Autodesk Inventor part; units mm, degrees
ref_plane "YZ Plane" through (0, 0, 0) normal (1, 0, 0) x (0, 1, 0)
ref_plane "XZ Plane" through (0, 0, 0) normal (0, 1, 0) x (-1, 0, 0)
ref_plane "XY Plane" through (0, 0, 0) normal (0, 0, 1) x (1, 0, 0)
sketch "Sketch1" plane through (0, 0, 0) normal (0, 0, 1) x (1, 0, 0)
  line L0 (0, 0) -> (100, 0)
  line L1 (100, 0) -> (100, 40)
  line L2 (100, 40) -> (0, 40)
  line L3 (0, 40) -> (0, 0)
  dimension "d0" = 100
  dimension "d1" = 40
extrude "Extrusion1" add sketch "Sketch1" along normal mid plane 40
sketch "Sketch2" plane through (100, 0, 20) normal (1, 0, 0) x (0, 0, -1)
  line L0 (40, 40) -> (0, 40)
  circle A0 centre (20, 20) radius 18
  point P0 (20, 0)
  dimension "d5" = 36
extrude "Extrusion2" add sketch "Sketch2" along normal blind 80
thread "Thread1"
chamfer "Chamfer1" distance 2 angle 45 1 edges at (180, 20, 18)
sketch "Sketch3" plane through (0, 0, 20) normal (0, 0, 1) x (1, 0, 0)
  line L0 (0, 0) -> (100, 0)
  line L1 (100, 40) -> (0, 40)
  circle A0 centre (20, 20) radius 7.5
  circle A1 centre (20, 20) radius 12.5
  line L2 (100, 0) -> (100, 40)
  dimension "d13" = 80
  dimension "d14" = 15
  dimension "d15" = 25
hole "Hole1" at (20, 20, 20) direction (0, 0, -1) diameter 15 end through all counterbore diameter 25 counterbore depth 5
fillet "Fillet1" radius 20 1 edges at (0, 40, 0)
fillet "Fillet2" radius 20 1 edges at (0, 0, 0)
sketch "Sketch9" plane through (100, 40, 20) normal (0, 1, 0) x (1, 0, 0)
  line L0 (0, 0) -> (-80, 0)
  line L1 (-28, 0) -> (-28, 39.5262)
  line L2 (0, 40) -> (0, 0)
  line L3 (-108, 28) -> (-28, 28)
  line L4 (-28, 28) -> (-28, 12)
  line L5 (-28, 12) -> (-108, 12)
  line L6 (-108, 12) -> (-108, 28)
  line L7 (-80, 40) -> (0, 40)
  circle A0 centre (-28, 20) radius 8
  point P0 (-100, 20)
  point P1 (-68, 12)
  point P2 (-28, 12)
  point P3 (-28, 28)
  dimension "d37" = 28
  dimension "d38" = 0
  dimension "d39" = 12
  dimension "d40" = 16
  dimension "d41" = 16
  dimension "d42" = 80
  dimension "d43" = 16
extrude "Extrusion5" cut sketch "Sketch9" against normal blind 40
sketch "Sketch12" plane through (0, 0, -20) normal (0, 0, -1) x (-1, 0, 0)
  line L0 (-20, 0) -> (-100, 0)
  circle A0 centre (-20, 20) radius 12.5
  circle A1 centre (-20, 20) radius 12.5
  point P0 (0, 0)
extrude "Extrusion6" cut sketch "Sketch12" against normal blind 5
properties part number "Partultimaparte"
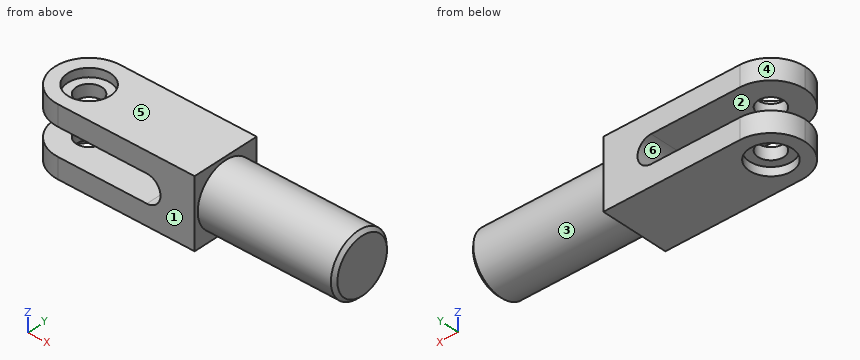
Geometry: final body of the model. Coordinates: model frame, mm. Face numbers are marked on the shaded views. A direction names the side the tool comes from. Coordinates: 2 decimals unless noted, no trailing zeros. Order: outer loops, then holes, each group sorted by start corner. A loop starts at its lowest first (then second) coordinate and runs counter-clockwise, first axis right, second up. Notation, with made-up numbers: M -11.75,-1 L 25.25,-1 A23 ccw 25.25,31 Z; hole C 80.5,87.25 d3. An arc over 180 degrees is marked long. Answer in a Markdown table with one row per item. Add a question column.
Q1. Reachability of the marked faces 1, 2 and 3 from +Z, -Z, +X, -X, +Y, -Y: full face, straight path, thin tool, end or side. Return the list, or none.
Q2. Section query A-A on x = 56. Return the cut outline in (y, z).
Q3. Section query B-B on z = 0. Return the cut outline in (x, y).
Q4. Contact query for flat-ended pins moving along their axis: P1, Ø6, axis at y = 8, z = -11.5, coming from the -X side; P2, Ø13.5, axis at x = 20, y = 20, coming from the -Z side (1 decimal); P3, Ø7.5, axis at x = 25, y = 14.5, coming from the -Z side; P4, Ø22.5, axis at x = 20, y = 20, coming from the +Z side. Output: stop coordinate, or through.
Q5. Line query: L1, parallel to Z at x = 67, y = 35; L2, parallel to Y at x = 20, z = 19; L3, parallel to X at y = 20, z = -10.5. Output: solid intervals per line, ascending.
Q6. Mould query, pull axis Z, two halves, no side actions, for the marked faces 4, 5 and 6. Classes: released by +Z, released by -Z, zero draft, split by the parting line, or undercut.
Q7. Section query D-D on x = 30.5. Return the cut outline in (y, z), and give its area (3 significant figures).
Q8. Section query C-C on y = 17. Count the separate pieces of the cut face and the enclosed holes in it, and give its area (3 significant figures).
Completed:
| question | item | result |
|---|---|---|
| 1 | face 1 | +Z, -Z, +X, -X, -Y |
| 1 | face 2 | -X, +Y, -Y |
| 1 | face 3 | +X |
| 2 | outline | M 0,-20 L 40,-20 L 40,-8 L 0,-8 Z; M 0,8 L 40,8 L 40,20 L 0,20 Z |
| 3 | outline | M 80,0 L 100,0 L 100,2 L 178,2 L 180,4 L 180,36 L 178,38 L 100,38 L 100,40 L 80,40 Z |
| 4 | P1 | stops at x = 2.14 |
| 4 | P2 | passes through |
| 4 | P3 | stops at z = -15 |
| 4 | P4 | stops at z = 15 |
| 5 | L1 | z = -20 to -8, 8 to 20 |
| 5 | L2 | y = 0 to 7.5, 32.5 to 40 |
| 5 | L3 | x = 0 to 12.5, 27.5 to 180 |
| 6 | face 4 | zero draft |
| 6 | face 5 | released by +Z |
| 6 | face 6 | undercut |
| 7 | outline | M 0,-20 L 13.22,-20 L 13.22,-15 L 26.78,-15 L 26.78,-20 L 40,-20 L 40,-8 L 0,-8 Z; M 0,8 L 40,8 L 40,20 L 26.78,20 L 26.78,15 L 13.22,15 L 13.22,20 L 0,20 Z |
| 7 | area | 824 mm2 |
| 8 | separate pieces | 3 |
| 8 | enclosed holes | 0 |
| 8 | area | 5,140 mm2 |
